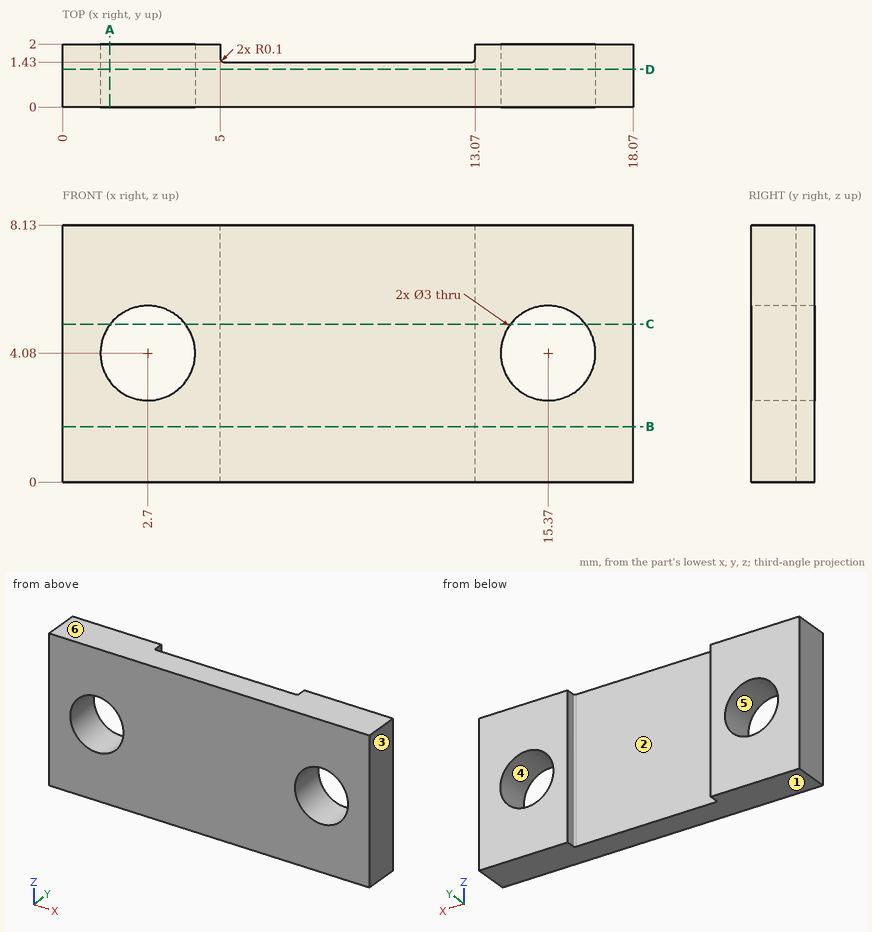
Could you check a few things on this drawing? It's one solid part, dimensions in mm from its lowest x, y, z. A direction names the side the tool comes from. Round coordinates to 2 decimals unless told otherwise and drop trailing zeros. Loops run counter-clockwise (first coordinate to the right, second up) from the corner with the lowest first, then second, coordinate; pieces in that order, holes last. Notation, with made-up numbers: (55, 56.5) -> (64, 56.5) arc R12 cw to (64, 75.5) -> close; hole circle Ø2 at (27.5, 74). An arc over 180 degrees is marked (long way). One line per item, written item: value. Start each with the question number.
1. If we mould it in two halves opening along Z, with no side actions, what happens to the marked faces 3, 4, 5 and 6? For each: pulls with the +Z half, pulls with the -Z half, needs draft (parallel to the pull), parting line crosses it, or undercut.
2. If we section it at C-C, the plane z = 5: Write out the boundary of the cut face in (x, y), then the cut area to 3 significant figures.
3. If I drill on probe 1 along X at (y, z) = (0.95, 4.08); probe 2 along Z at (x, y) = (15.37, 1.2); probe 3 along X at (y, z) = (1.6, 3.25), over which ranges is the centre line in solid material (lowest first)?
4. If we section it at D-D, the plane y = 1.2: Write out the boundary of the cut face in (x, z), then the cut area to 3 significant figures.
5. If we section it at A-A, the plane x = 1.5: Write out the boundary of the cut face in (y, z), then the cut area to 3 significant figures.
6. For the marked faces 1 and 2, which set-ups out of +Z, -Z, +X, -X, +Y, -Y let a thin tool reach every point of the face, with its end or its side?
7. For pin 1 (2.5 mm diameter, centred on x = 9, z = 3.5, fed in from +Y); pin 2 (0.5 mm diameter, centred on y = 2, z = 4.5, fed in from -X), each with a flat end and sliding along its axis, tell me the tip position at first contact or that it passes through.
8. If we section it at B-B, the plane z = 1.75: Write out the boundary of the cut face in (x, y).
Calculated:
1. face 3: needs draft
1. face 4: undercut
1. face 5: undercut
1. face 6: pulls with the +Z half
2. outline: (0, 0) -> (1.52, 0) -> (1.52, 2) -> (0, 2) -> close; (3.88, 0) -> (14.19, 0) -> (14.19, 2) -> (13.07, 2) -> (13.07, 1.53) arc R0.1 cw to (12.97, 1.43) -> (5.1, 1.43) arc R0.1 cw to (5, 1.53) -> (5, 2) -> (3.88, 2) -> close; (16.55, 0) -> (18.07, 0) -> (18.07, 2) -> (16.55, 2) -> close
2. area: 22.1 mm²
3. probe 1: x = 0 to 1.2, 4.2 to 13.87, 16.87 to 18.07
3. probe 2: z = 0 to 2.58, 5.58 to 8.13
3. probe 3: x = 0 to 1.45, 3.95 to 5, 13.07 to 14.12, 16.62 to 18.07
4. outline: (0, 0) -> (18.07, 0) -> (18.07, 8.13) -> (0, 8.13) -> close; hole circle Ø3 at (2.7, 4.08); hole circle Ø3 at (15.37, 4.08)
4. area: 133 mm²
5. outline: (0, 0) -> (2, 0) -> (2, 3.18) -> (0, 3.18) -> close; (0, 4.98) -> (2, 4.98) -> (2, 8.13) -> (0, 8.13) -> close
5. area: 12.7 mm²
6. face 1: -Z, +X, -X, +Y, -Y
6. face 2: +Z, -Z, +Y
7. pin 1: stops at y = 1.43
7. pin 2: stops at x = 0
8. outline: (0, 0) -> (18.07, 0) -> (18.07, 2) -> (13.07, 2) -> (13.07, 1.53) arc R0.1 cw to (12.97, 1.43) -> (5.1, 1.43) arc R0.1 cw to (5, 1.53) -> (5, 2) -> (0, 2) -> close
